Check sheet for the drawn part. Datum: minimum x, y, z corner. Units: mm. Round coordinates to 2 decimals unless told otherwise and drop trailing zeros. Write each loop counter-clockwise with the first axis right and the second up, starting at its lowest first coordinate (ties: lowest second). Pieces come first, ordered by that corner, then holes. Notation, with made-up numbers: M 83.25,7.5 L 110.25,7.5 A15 cw 110.25,12.5 Z; hole C 10.5,50.5 d7. An arc over 180 degrees is marked long. One line per item, written item: value. Start each with the question number.
Item 1: Gauge pin test, flat end, axial feed: pin 1 (2.5 mm diameter, centred on x = 39.475, y = 10, fed in from +Z). Record the tip position at first contact, or that the pin passes through.
Item 2: Section check A-A, the plane x = 218.06. Record the cut outline in (y, z) (1 decimal).
Item 3: Section check B-B, the plane y = 10. Record the cut outline in (x, z) (1 decimal).
Item 4: Thickness scan on probe 1 along X at (y, z) = (11.25, 1.1) (1 decimal); probe 2 along X at (y, z) = (9, 2.7) (1 decimal); probe 3 along Y at (x, z) = (218.06, 1.2). Record the ranges inside material, lowest first. Write a range as from..to.
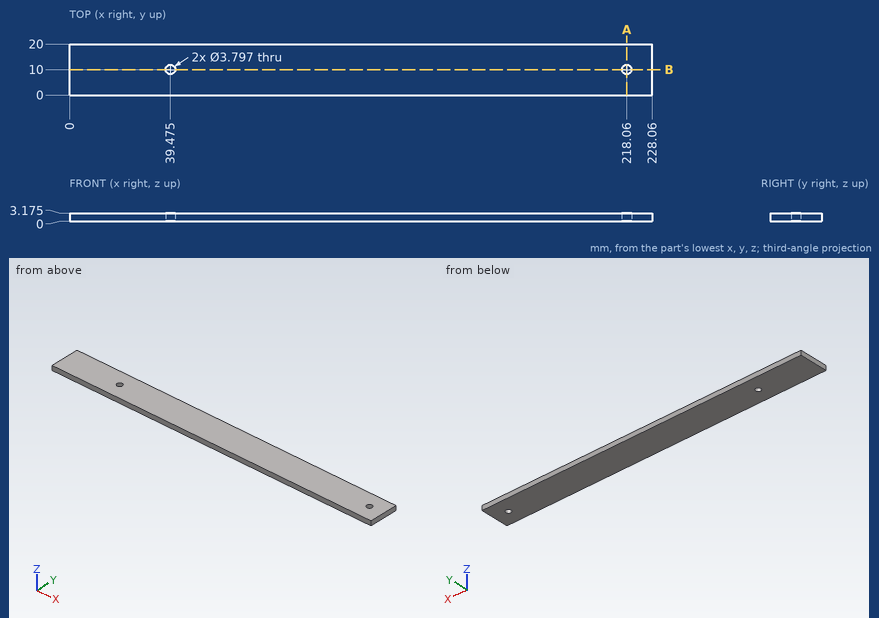
Response values:
1. pin 1: passes through
2. outline: M 0,0 L 8.1,0 L 8.1,3.2 L 0,3.2 Z; M 11.9,0 L 20,0 L 20,3.2 L 11.9,3.2 Z
3. outline: M 0,0 L 37.6,0 L 37.6,3.2 L 0,3.2 Z; M 41.4,0 L 216.2,0 L 216.2,3.2 L 41.4,3.2 Z; M 220,0 L 228.1,0 L 228.1,3.2 L 220,3.2 Z
4. probe 1: x = 0..38, 40.9..216.6, 219.5..228.1
4. probe 2: x = 0..37.9, 41.1..216.4, 219.7..228.1
4. probe 3: y = 0..8.1, 11.9..20
